The model under review builds one solid part; all positions refer to its coordinate system, in mm. Give positions to 0.01 mm unless a question says otherwise; leave off trailing zeros. Loops run counter-clockwise (first coordinate to the right, second up) from the corner with the lowest first, then second, coordinate; pieces in that order, holes last. Notation, with made-up numbers: M 66,9.25 L 78,9.25 A17 ccw 78,22.25 Z; hole C -28,66.25 d7. An arc over 180 degrees is marked long. Write item = value, one per line. Start each with the question number.
1. We need section B-B on y = 4.5. Count the separate pieces of the cut face and the enclosed holes in it, then the cut area to 3 significant figures.
2. We need section D-D on x = 8. Give the boundary of the cut face in (y, z), then the cut area to 3 significant figures.
3. We need section C-C on z = 80.5. Give the boundary of the cut face in (x, y) (3 decimals).
4. We need section A-A on x = 0. Give the boundary of the cut face in (y, z) (3 decimals).
5. Wall thickness on line 1 along X through (y, z) = (-0.5, 103); line 2 along Y through (x, z) = (0, 89.5) (3 decimals); line 3 along Z through (x, y) = (-9, 6.5): over which ranges is each line inside the solid? List them lowest first. Write a range as from..to.
6. For pin 1 (4 mm diameter, centred on y = 2.5, z = 82.5, fed in from -X); pin 2 (10 mm diameter, centred on x = -14.5, z = 19, fed in from -Y); pin 3 (6 mm diameter, centred on x = -9, z = 17, fed in from +Y); pin 4 (3 mm diameter, centred on x = -1, y = 8.5, fed in from +Z), all flat-tipped, find the tip position at first contact; note any pin that passes through.
from build123d import *

# Parameters (mm, degrees)
F0_R          = 12.7
F0_R_2        = 9.525
F1_DEPTH      = 158.98622
F2_R          = 4.7625
F2_R_2        = 3.175
F3_DEPTH      = 6.35
F3_DEPTH_BACK = 6.35


with BuildPart() as f1:
    # F0 (on Top) → F1 (new body)
    with BuildSketch(Plane.XY):
        Circle(F0_R)
        Circle(F0_R_2, mode=Mode.SUBTRACT)
    extrude(amount=F1_DEPTH)

    # F2 (on Front) → F3 (join, two sides)
    with BuildSketch(Plane.XZ) as f3_sk:
        with Locations((-17.27381, 3.554616)):
            Circle(F2_R)
        with Locations((-17.27381, 3.554616)):
            Circle(F2_R_2, mode=Mode.SUBTRACT)
    extrude(amount=F3_DEPTH)
    extrude(f3_sk.sketch, amount=-F3_DEPTH_BACK)


solid = f1.part
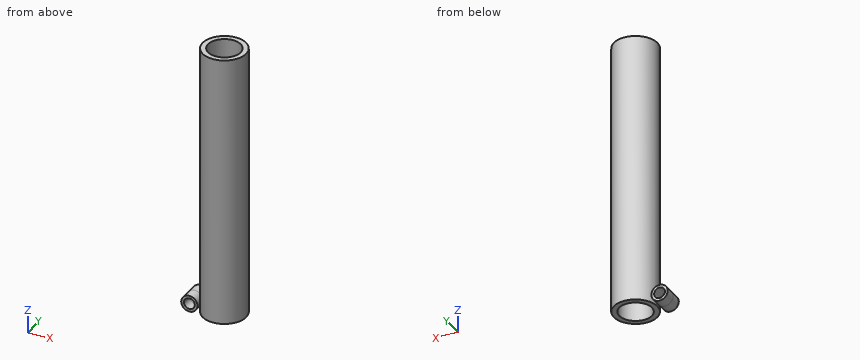
Final values:
q1.separate_pieces = 3
q1.enclosed_holes = 1
q1.area = 1,150 mm²
q2.outline = M -9.86,0 L -5.17,0 L -5.17,158.99 L -9.86,158.99 Z; M 5.17,0 L 9.86,0 L 9.86,158.99 L 5.17,158.99 Z
q2.area = 1,490 mm²
q3.outline = C 0,0 d25.4; hole C 0,0 d19.05
q4.outline = M -12.7,0 L -9.525,0 L -9.525,158.986 L -12.7,158.986 Z; M 9.525,0 L 12.7,0 L 12.7,158.986 L 9.525,158.986 Z
q5.line_1 = -12.69..-9.51, 9.51..12.69
q5.line_2 = -12.7..-9.525, 9.525..12.7
q5.line_3 = 0..158.99
q6.pin_1 = -12.69
q6.pin_2 = -8.43
q6.pin_3 = 11.19
q6.pin_4 = 158.99
